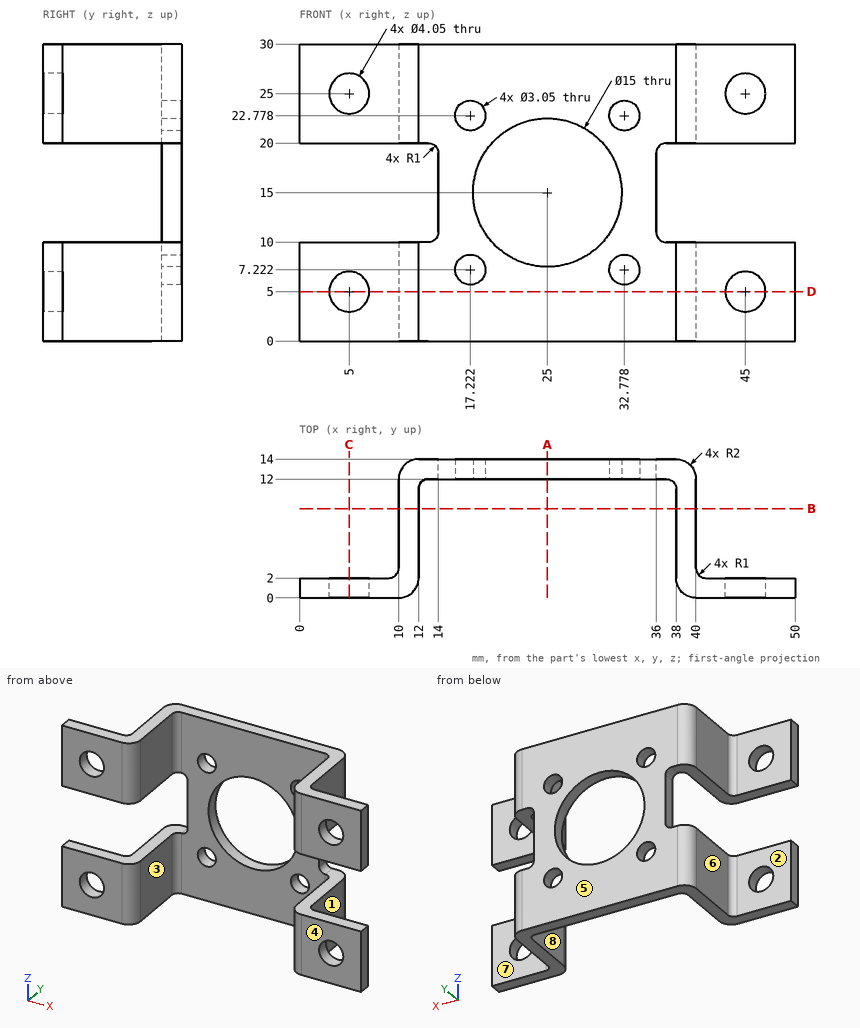
Design review of the part shown in the three views and the two pictorial views. Dimensions are in mm from the part's minimum x, y and z. A direction names the side the tool comes from. Give positions to 0.01 mm unless a question says otherwise; leave off trailing zeros. Write each loop counter-clockwise with the first axis right and the second up, starting at its lowest first coordinate (ties: lowest second). Pieces come first, ordered by that corner, then holes. Notation, with made-up numbers: M 75.5,7.25 L 99.5,7.25 A4 cw 99.5,13.25 Z; hole C -18.75,69 d9. An arc over 180 degrees is marked long. Answer as CSV lines item,"result".
1. For the marked faces 4, 5, 6, 7 and 8, list the 3-axis set-ups (+Z, -Z, +X, -X, +Y, -Y) from which the entire face can be reached by the end or side of a thin tool; tool diameter is ignored.
Findings:
face 4,"+Z, -Z, +X, -X, -Y"
face 5,"+Z, -Z, +X, -X, +Y"
face 6,"+Z, -Z, -X, +Y"
face 7,"+Z, -Z, +X, +Y"
face 8,"+Z, -Z, -Y"
2. Draft analysis for pull direction X (two halves, no side actions). For the marked faces 1, 2 and 3, state which applies: +X half, -X half, draft (parallel to the pull), parting line (faces both ways), or undercut.
Findings:
face 1,"+X half"
face 2,"draft"
face 3,"undercut"
3. Wall thickness on line 1 (X direction, y = 4, z = 27.75); line 2 (X direction, y = 1.35, z = 25) (1 decimal); line 3 (X direction, y = 13.4, z = 15): over which ranges is each line inside the solid? List them lowest first.
Findings:
line 1,"x = 10 to 12, 38 to 40"
line 2,"x = 0 to 3, 7 to 11.9, 38.1 to 43, 47 to 50"
line 3,"x = 14 to 17.5, 32.5 to 36"
4. For pin 1 (7 mm diameter, centred on y = 7.5, z = 6.5, fed in from -X); pin 2 (2.5 mm diameter, centred on x = 32.78, z = 7.22, fed in from +Y); pin 3 (2 mm diameter, centred on x = 43.5, z = 20, fed in from +Y); pin 4 (4.5 mm diameter, centred on y = 8.5, z = 2.5, fed in from +X), all flat-tipped, find the tip position at first contact; note any pin that passes through.
Findings:
pin 1,"stops at x = 10"
pin 2,"passes through"
pin 3,"stops at y = 2"
pin 4,"stops at x = 40"
5. Consider section B-B, the plane y = 9. Write out the cut boundary in (x, z).
Findings:
outline,"M 10,0 L 12,0 L 12,10 L 10,10 Z; M 10,20 L 12,20 L 12,30 L 10,30 Z; M 38,0 L 40,0 L 40,10 L 38,10 Z; M 38,20 L 40,20 L 40,30 L 38,30 Z"
6. Consider section D-D, the plane z = 5. Write out the cut boundary in (x, y) (3 decimals).
Findings:
outline,"M 0,0 L 2.975,0 L 2.975,2 L 0,2 Z; M 7.025,0 L 10,0 A2 ccw 12,2 L 12,11 A1 cw 13,12 L 37,12 A1 cw 38,11 L 38,2 A2 ccw 40,0 L 42.975,0 L 42.975,2 L 41,2 A1 cw 40,3 L 40,12 A2 ccw 38,14 L 12,14 A2 ccw 10,12 L 10,3 A1 cw 9,2 L 7.025,2 Z; M 47.025,0 L 50,0 L 50,2 L 47.025,2 Z"
7. Consider section C-C, the plane x = 5. Write out the cut boundary in (y, z) (3 decimals), then the cut area to 3 significant figures.
Findings:
outline,"M 0,0 L 2,0 L 2,2.975 L 0,2.975 Z; M 0,7.025 L 2,7.025 L 2,10 L 0,10 Z; M 0,20 L 2,20 L 2,22.975 L 0,22.975 Z; M 0,27.025 L 2,27.025 L 2,30 L 0,30 Z"
area,"23.8 mm2"
8. Consider section A-A, the plane x = 25. Write out the cut boundary in (y, z).
Findings:
outline,"M 12,0 L 14,0 L 14,7.5 L 12,7.5 Z; M 12,22.5 L 14,22.5 L 14,30 L 12,30 Z"
